from build123d import *

# Parameters (mm, degrees)
F1_DEPTH       = 1096.09636
F3_DEPTH       = 254.001
F5_D           = 9
F5_DEPTH       = 10
F5_CBORE_D     = 12
F5_CBORE_DEPTH = 1.5


with BuildPart() as f1:
    # F0 (on Front) → F1 (new body)
    with BuildSketch(Plane.XZ):
        with BuildLine():
            Line((-41.275, 0), (-9.525, 0))
            ThreePointArc((-9.525, 0), (-2.789808, 2.789808), (0, 9.525))
            Line((0, 9.525), (0, 244.475))
            ThreePointArc((0, 244.475), (-2.789808, 251.210192), (-9.525, 254))
            Line((-9.525, 254), (-41.275, 254))
            ThreePointArc((-41.275, 254), (-48.010192, 251.210192), (-50.8, 244.475))
            Line((-50.8, 244.475), (-50.8, 9.525))
            ThreePointArc((-50.8, 9.525), (-48.010192, 2.789808), (-41.275, 0))
        make_face()
        with BuildLine():
            ThreePointArc((-46.0502, 244.5004), (-44.659016, 247.859016), (-41.3004, 249.2502))
            Line((-41.3004, 249.2502), (-9.4996, 249.2502))
            ThreePointArc((-9.4996, 249.2502), (-6.140984, 247.859016), (-4.7498, 244.5004))
            Line((-4.7498, 244.5004), (-4.7498, 9.4996))
            ThreePointArc((-4.7498, 9.4996), (-6.140984, 6.140984), (-9.4996, 4.7498))
            Line((-9.4996, 4.7498), (-41.3004, 4.7498))
            ThreePointArc((-41.3004, 4.7498), (-44.659016, 6.140984), (-46.0502, 9.4996))
            Line((-46.0502, 9.4996), (-46.0502, 244.5004))
        make_face(mode=Mode.SUBTRACT)
    extrude(amount=F1_DEPTH)

    # F2 (on face) → F3 (cut, through all)
    with BuildSketch(Plane.XY.offset(254)):
        Polygon((0, 0), (-50.8, 0), (0, -50.8), align=None)
        Polygon((0, -1045.29636), (-50.8, -1096.09636), (0, -1096.09636), align=None)
    extrude(amount=-F3_DEPTH, mode=Mode.SUBTRACT)

    # F5
    with Locations(Plane.YZ):
        with Locations((-892.43736, 188.628289), (-892.43736, 145.628289), (-892.43736, 102.628289), (-892.43736, 59.628289), (-892.43736, 16.628289), (-609.26236, 188.628289), (-609.26236, 145.628289), (-609.26236, 102.628289), (-609.26236, 59.628289), (-609.26236, 16.628289), (-399.85, 188.628509), (-399.85, 145.628289), (-399.85, 102.628289), (-399.85, 59.628289), (-399.85, 16.628289), (-116.675, 188.628509), (-116.675, 145.628289), (-116.675, 102.628289), (-116.675, 59.628289), (-116.675, 16.628289)):
            CounterBoreHole(F5_D / 2, F5_CBORE_D / 2, F5_CBORE_DEPTH, depth=F5_DEPTH)


solid = f1.part
Here's how the part is built. I have some questions about the finished solid (model axes, mm). A direction names the side the tool comes from. Coordinates: 2 decimals unless noted, no trailing zeros. Loops run counter-clockwise (first coordinate to the right, second up) from the corner with the lowest first, then second, coordinate; pieces in that order, holes last. Notation, with made-up numbers: (36, 17.25) -> (44, 17.25) arc R33 ccw to (44, 46.25) -> close; hole circle Ø11 at (70, 55). An arc over 180 degrees is marked (long way). Use one line per item in the form item = value. Start each with the question number.
(1) If we section it at A-A (y = -498.5): Please give me the cut outline in (x, z) (3 decimals), then the cut area to 3 significant figures.
(2) On a 3-axis mill with a long thin cutter (end or side, diameter ignored), from which of +Z, -Z, +X, -X, +Y, -Y can I reach the whole of each face in a straight line? I mean faces 1 (the face through (-46.2, -4.6, 137)), 2 (the face through (-46.05, -540, 125)). Say none if no direction works.
(3) We'd pull the mould along Z, two halves only. Please class faces 3 (the face through (-50.8, -540, 129)), 4 (the face through (-26, -541, 0)), 5 (the face through (-26, -541, 249.25)): pulls with the +Z half, pulls with the -Z half, needs draft (parallel to the pull), parting line crosses it, or undercut.
(4) If we section it at B-B (x = -27): Please give me the cut outline in (y, z).
(5) Will these pins go through, and if not, where does the flat tip stop? pin 1 (8 mm diameter, centred on y = -475, z = 143, fed in from +X); pin 2 (3.5 mm diameter, centred on y = -892, z = 146.5, fed in from +X); pin 3 (3.5 mm diameter, centred on y = -889.5, z = 15.5, fed in from +X).
(6) Please list where these lines run through material, in increasing order: line 1 along Z through (x, y) = (-15, -165.5); line 2 along X through (y, z) = (-90.5, 31); line 3 along Z through (x, y) = (-2.95, -399.85).
Verdict:
q1.outline = (-50.8, 9.525) arc R9.525 ccw to (-41.275, 0) -> (-9.525, 0) arc R9.525 ccw to (0, 9.525) -> (0, 244.475) arc R9.525 ccw to (-9.525, 254) -> (-41.275, 254) arc R9.525 ccw to (-50.8, 244.475) -> close; hole (-46.05, 9.5) arc R4.75 ccw to (-41.3, 4.75) -> (-9.5, 4.75) arc R4.75 ccw to (-4.75, 9.5) -> (-4.75, 244.5) arc R4.75 ccw to (-9.5, 249.25) -> (-41.3, 249.25) arc R4.75 ccw to (-46.05, 244.5) -> close
q1.area = 2,750 mm²
q2.face_1 = +Z, -Z, +X, +Y
q2.face_2 = +Y, -Y
q3.face_3 = needs draft
q3.face_4 = pulls with the -Z half
q3.face_5 = undercut
q4.outline = (-1072.3, 0) -> (-23.8, 0) -> (-23.8, 4.75) -> (-1072.3, 4.75) -> close; (-1072.3, 249.25) -> (-23.8, 249.25) -> (-23.8, 254) -> (-1072.3, 254) -> close
q5.pin_1 = 0
q5.pin_2 = -46.05
q5.pin_3 = -1.5
q6.line_1 = 0 to 4.75, 249.25 to 254
q6.line_2 = -50.8 to -46.05, -4.75 to 0
q6.line_3 = 2.63 to 12.13, 21.13 to 55.13, 64.13 to 98.13, 107.13 to 141.13, 150.13 to 184.13, 193.13 to 251.37
